```python
from build123d import *

# Parameters (mm, degrees)
SKETCH1_W               = 72.263
SKETCH1_H               = 44.45
BOSS_EXTRUDE1_DEPTH     = 12.7
CUT_EXTRUDE1_DEPTH      = 59.673484576
SKETCH3_W               = 44.45
SKETCH3_H               = 25.4
BOSS_EXTRUDE2_DEPTH     = 10.16
F_1_4_CLEARANCE_HOLE1_D = 6.5278
FILLET8_R               = 1.27


with BuildPart() as part:
    # Sketch1 → Boss-Extrude1 (new, symmetric)
    with BuildSketch(Plane(origin=(0, 0, 0), x_dir=(1, 0, 0), z_dir=(0, 1, 0))):
        Rectangle(SKETCH1_W, SKETCH1_H)
    extrude(amount=BOSS_EXTRUDE1_DEPTH, both=True)

    # Sketch2 → Cut-Extrude1 (cut, through all)
    with BuildSketch(Plane.XY.offset(22.225)):
        with BuildLine():
            Line((-16.002, -12.7), (16.002, -12.7))
            ThreePointArc((16.002, -12.7), (0, 3.302), (-16.002, -12.7))
        make_face()
    extrude(amount=-CUT_EXTRUDE1_DEPTH, mode=Mode.SUBTRACT)

    # Sketch3 → Boss-Extrude2 (add)
    with BuildSketch(Plane.ZY.offset(36.1315)):
        Rectangle(SKETCH3_W, SKETCH3_H)
    extrude(amount=BOSS_EXTRUDE2_DEPTH)

    # 1/4 Clearance Hole1 (through all)
    with Locations(Plane(origin=(-39.37, -12.7, 15.875), x_dir=(0, 0, -1), z_dir=(0, -1, 0))):
        with Locations((0, 0), (0, 68.58), (31.75, 68.58), (31.75, 0)):
            Hole(F_1_4_CLEARANCE_HOLE1_D / 2)

    # Fillet8
    fillet8_edges = [part.edges().sort_by_distance(p)[0] for p in [
        (-5.08, 12.7, 22.225),
        (-46.2915, 0, -22.225),
        (-46.2915, 0, 22.225),
        (-46.2915, 12.7, 0),
        (36.1315, 12.7, 0),
        (-5.08, 12.7, -22.225),
        (36.1315, 0, 22.225),
        (36.1315, 0, -22.225),
    ]]
    fillet(fillet8_edges, radius=FILLET8_R)


solid = part.part
```
Could you check a few things on this model? Use its own coordinates, in mm. Coordinates: 2 decimals unless noted, no trailing zeros. Order: outer loops, then holes, each group sorted by start corner. A loop starts at its lowest first (then second) coordinate and runs counter-clockwise, first axis right, second up. Notation, with made-up numbers: M 10.5,67 L 30.5,67 A24 ccw 30.5,90 Z; hole C 33,12 d10. An arc over 180 degrees is marked long. Use one line per item in the form item = value. Start each with the question number.
1. Suppose I cut it at B-B on x = 29.21. Write out the boundary of the cut face in (y, z) (3 decimals).
2. For pin 1 (8.5 mm diameter, centred on x = 29.21, z = -15.875, fed in from +Y); pin 2 (6 mm diameter, centred on x = 29.21, z = 15.875, fed in from -Y), each with a flat end and sliding along its axis, tell me the tip position at first contact or that it passes through.
3. Suppose I cut it at C-C on z = 16. Write out the boundary of the cut face in (x, y).
4. Suppose I cut it at A-A on y = -9. Write out the boundary of the cut face in (x, z) (1 decimal).
5. Suppose I cut it at D-D on z = -10.5. Write out the boundary of the cut face in (x, y), then the cut area to 3 significant figures.
6. Please list where these lines run through material, in increasing order: line 1 (Z direction, x = 29.5, y = 8) (3 decimals); line 2 (X direction, y = -5.5, z = 15); line 3 (X direction, y = -9.5, z = -14).
7. We'd pull the mould along X, two halves only. Please class faces 1 (the flat face through (26, -12.7, 0)), 2 (the cylindrical face through (26.024, 0.178, -16.583)), 3 (the flat face through (-46.292, 0, 0)), 4 (the flat face through (36.132, 0, 0)): +X half, -X half, draft (parallel to the pull), parting line (faces both ways), or undercut.
Geometry says:
q1.outline = M -12.7,-22.225 L 11.43,-22.225 A1.27 ccw 12.7,-20.955 L 12.7,-19.139 L -12.7,-19.139 Z; M -12.7,-12.611 L 12.7,-12.611 L 12.7,12.611 L -12.7,12.611 Z; M -12.7,19.139 L 12.7,19.139 L 12.7,20.955 A1.27 ccw 11.43,22.225 L -12.7,22.225 Z
q2.pin_1 = 12.7
q2.pin_2 = through
q3.outline = M -46.29,-12.7 L -42.63,-12.7 L -42.63,12.7 L -45.02,12.7 A1.27 ccw -46.29,11.43 Z; M -36.11,-12.7 L -16,-12.7 A16 cw 16,-12.7 L 25.95,-12.7 L 25.95,12.7 L -36.11,12.7 Z; M 32.47,-12.7 L 36.13,-12.7 L 36.13,11.43 A1.27 ccw 34.86,12.7 L 32.47,12.7 Z
q4.outline = M -46.3,-21 A1.3 ccw -45,-22.2 L -15.6,-22.2 L -15.6,22.2 L -45,22.2 A1.3 ccw -46.3,21 Z; M 15.6,-22.2 L 34.9,-22.2 A1.3 ccw 36.1,-21 L 36.1,21 A1.3 ccw 34.9,22.2 L 15.6,22.2 Z; hole C -39.4,-15.9 d6.5; hole C -39.4,15.9 d6.5; hole C 29.2,-15.9 d6.5; hole C 29.2,15.9 d6.5
q5.outline = M -46.29,-12.7 L -16,-12.7 A16 cw 16,-12.7 L 36.13,-12.7 L 36.13,11.43 A1.27 ccw 34.86,12.7 L -45.02,12.7 A1.27 ccw -46.29,11.43 Z
q5.area = 1,690 mm^2
q6.line_1 = -22.225 to -19.126, -12.624 to 12.624, 19.126 to 22.225
q6.line_2 = -46.29 to -42.51, -36.23 to -14.29, 14.29 to 26.07, 32.35 to 36.13
q6.line_3 = -46.29 to -42.04, -36.7 to -15.68, 15.68 to 26.54, 31.88 to 36.13
q7.face_1 = draft
q7.face_2 = undercut
q7.face_3 = -X half
q7.face_4 = +X half
